```python
from build123d import *

# Parameters (mm, degrees)
SKETCH1_W                               = 270
SKETCH1_H                               = 30
BOSS_EXTRUDE1_DEPTH                     = 13
CBORE_FOR_M8_HEX_HEAD_BOLT1_D           = 9
CBORE_FOR_M8_HEX_HEAD_BOLT1_DEPTH       = 15
CBORE_FOR_M8_HEX_HEAD_BOLT1_CBORE_D     = 18.011
CBORE_FOR_M8_HEX_HEAD_BOLT1_CBORE_DEPTH = 5.3
CBORE_FOR_M8_HEX_HEAD_BOLT1_TIP         = 2.703872786


with BuildPart() as part:
    # Sketch1 → Boss-Extrude1 (new body)
    with BuildSketch(Plane(origin=(0, 0, 0), x_dir=(1, 0, 0), z_dir=(0, 1, 0))):
        Rectangle(SKETCH1_W, SKETCH1_H)
    extrude(amount=BOSS_EXTRUDE1_DEPTH)

    # CBORE for M8 Hex Head Bolt1
    with Locations(Plane(origin=(-105, 13, 0), x_dir=(0, 0, 1), z_dir=(0, 1, 0))):
        with Locations((0, 0), (0, 210)):
            CounterBoreHole(CBORE_FOR_M8_HEX_HEAD_BOLT1_D / 2, CBORE_FOR_M8_HEX_HEAD_BOLT1_CBORE_D / 2, CBORE_FOR_M8_HEX_HEAD_BOLT1_CBORE_DEPTH, depth=CBORE_FOR_M8_HEX_HEAD_BOLT1_DEPTH)
            with Locations((0, 0, -(CBORE_FOR_M8_HEX_HEAD_BOLT1_DEPTH + CBORE_FOR_M8_HEX_HEAD_BOLT1_TIP / 2))):  # 118° drill point
                Cone(0, CBORE_FOR_M8_HEX_HEAD_BOLT1_D / 2, CBORE_FOR_M8_HEX_HEAD_BOLT1_TIP, mode=Mode.SUBTRACT)


solid = part.part
```
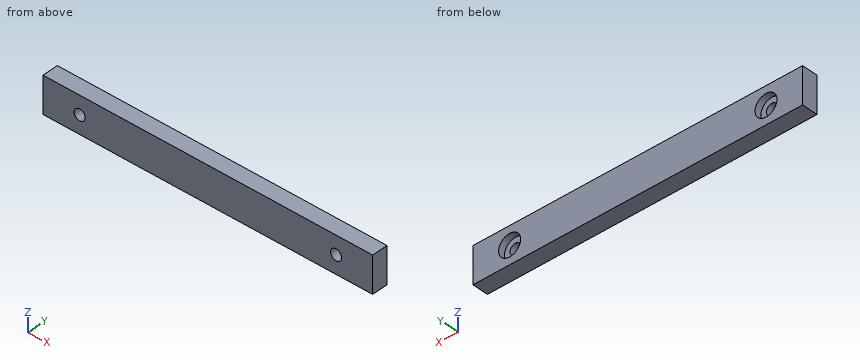
Can you work these out from the model? Positions are in its coordinate system, mm. Round coordinates to 2 decimals unless told otherwise and drop trailing zeros. Loops run counter-clockwise (first coordinate to the right, second up) from the corner with the lowest first, then second, coordinate; pieces in that order, holes last.
Item 1: Suppose I cut it at A-A, the plane z = 0. Write out the boundary of the cut face in (x, y), then the cut area to 3 significant figures.
Item 2: Suppose I cut it at B-B, the plane x = -105. Write out the boundary of the cut face in (y, z).
Item 3: Please list where these lines run through material, in increasing order: L1, parallel to X at y = 5.75, z = 0; L2, parallel to X at y = 9.65, z = 0; L3, parallel to Y at x = 111.5, z = 1.5.
Item 4: Suppose I cut it at C-C, the plane y = 5.25. Write out the boundary of the cut face in (x, z).
Item 5: Will these pins go through, and if not, where does the flat tip stop? pin 1 Ø11 at (x, z) = (105, 0) entering from +Y; pin 2 Ø5.5 at (x, z) = (-106, -0.5) entering from +Y.
Reported:
1. outline: (-135, 0) - (-109.5, 0) - (-109.5, 7.7) - (-114.01, 7.7) - (-114.01, 13) - (-135, 13) - close; (-100.5, 0) - (100.5, 0) - (100.5, 7.7) - (95.99, 7.7) - (95.99, 13) - (-95.99, 13) - (-95.99, 7.7) - (-100.5, 7.7) - close; (109.5, 0) - (135, 0) - (135, 13) - (114.01, 13) - (114.01, 7.7) - (109.5, 7.7) - close
1. area: 3,180 mm2
2. outline: (0, -15) - (13, -15) - (13, -9.01) - (7.7, -9.01) - (7.7, -4.5) - (0, -4.5) - close; (0, 4.5) - (7.7, 4.5) - (7.7, 9.01) - (13, 9.01) - (13, 15) - (0, 15) - close
3. L1: x = -135 to -109.5, -100.5 to 100.5, 109.5 to 135
3. L2: x = -135 to -114.01, -95.99 to 95.99, 114.01 to 135
3. L3: y = 0 to 7.7
4. outline: (-135, -15) - (135, -15) - (135, 15) - (-135, 15) - close; hole circle Ø9 at (-105, 0); hole circle Ø9 at (105, 0)
5. pin 1: stops at y = 7.7
5. pin 2: passes through
